The model under review builds one solid part; all positions refer to its coordinate system, in mm. A direction names the side the tool comes from. Round coordinates to 2 decimals unless told otherwise and drop trailing zeros. Write each loop counter-clockwise with the first axis right and the second up, starting at its lowest first coordinate (ties: lowest second). Pieces come first, ordered by that corner, then holes. Notation, with made-up numbers: (61, -36) -> (114, -36) arc R10 ccw to (114, -30) -> close; hole circle Ø11 at (-1.5, 40.5). An arc over 180 degrees is marked (long way). Answer as a JSON object with one key per item and string values. Group by question number.
1) We need section B-B, the plane y = 40.5. Write out the cut boundary in (x, z), then the cut area to 3 significant figures.
2) Mouldability with a two-part tool opening along Y and no side actions: class faces 1 (the flat face through (88, 57.098, 3)), 2 (the flat face through (68, 55, 6)), 3 (the flat face through (107.925, 21.234, 2.958)) as pulls with the +Y half, pulls with the -Y half, needs draft (parallel to the pull), parting line crosses it, or undercut.
3) We need section C-C, the plane z = 3.4. Count the separate pieces of the cut face and the enclosed holes in it, then the cut area to 3 significant figures.
4) Machinability: for faces 4 (the flat face through (27.52, 20.93, 2.96)), 5 (the flat face through (93.83, 73.414, 2.958)), which of the approach directions +Z, -Z, +X, -X, +Y, -Y give a long, thin tool a straight path to every point of the face, cutting with its end or side? Answer none if there is none.
5) To check wall thickness, follow probe 1 along X at (y, z) = (78.5, 3.3); probe 2 along X at (y, z) = (69, 2.8); probe 3 along X at (y, z) = (71, 1.3). State the ranges of each line that lie inside material, in increasing order. Write a range as [from, to].
6) We need section A-A, the plane y = 54. Write out the cut boundary in (x, z).
7) Insertion check: pin 1 Ø1 at (y, z) = (51, 4) entering from -X; pin 2 Ø2.5 at (y, z) = (67.5, 2) entering from -X; pin 3 Ø1.6 at (y, z) = (66.5, 3.5) entering from +X. Each pin has a flat end and moves straight along its axis. Give the tip position at first contact, or say it passes through.
8) We need section D-D, the plane y = 75. Write out the cut boundary in (x, z), then the cut area to 3 significant figures.
from build123d import *

# Parameters (mm, degrees)
MODEL_R             = 3
MODEL_R_2           = 1.5
MODEL_W             = 5.5
MODEL_H             = 5.25
BOSS_EXTRUDE1_DEPTH = 6


with BuildPart() as part:
    # Model → Boss-Extrude1 (new body)
    with BuildSketch(Plane.XY):
        with BuildLine():
            Line((97.092556574, 10.401311798), (38.049140345, 10.401311798))
            Line((38.049140345, 10.401311798), (16.682633066, 31.767819077))
            Line((16.682633066, 31.767819077), (16.576099155, 46.615832828))
            ThreePointArc((16.576099155, 46.615832828), (67.57084846, 98.347641115), (118.565597764, 46.615832828))
            Line((118.565597764, 46.615832828), (118.459063854, 31.767819077))
            Line((118.459063854, 31.767819077), (97.092556574, 10.401311798))
        make_face()
        with Locations((67.57084846, 47.347641115)):
            Circle(MODEL_R, mode=Mode.SUBTRACT)
        with Locations((67.57084846, 57.347641115)):
            Circle(MODEL_R_2, mode=Mode.SUBTRACT)
        with Locations((77.57084846, 47.347641115)):
            Circle(MODEL_R_2, mode=Mode.SUBTRACT)
        with Locations((67.57084846, 37.347641115)):
            Circle(MODEL_R_2, mode=Mode.SUBTRACT)
        with Locations((57.57084846, 47.347641115)):
            Circle(MODEL_R_2, mode=Mode.SUBTRACT)
        Polygon((45.296984853, 69.621504723), (52.191275969, 76.515795839), (48.302188673, 80.404883136), (34.513606439, 66.616300902), (38.402693736, 62.727213606), align=None, mode=Mode.SUBTRACT)
        Polygon((45.296984853, 25.073777508), (52.191275969, 18.179486391), (48.302188673, 14.290399095), (34.513606439, 28.078981328), (38.402693736, 31.968068624), align=None, mode=Mode.SUBTRACT)
        Polygon((89.844712067, 69.621504723), (96.739003184, 62.727213606), (100.62809048, 66.616300902), (86.839508247, 80.404883136), (82.950420951, 76.515795839), align=None, mode=Mode.SUBTRACT)
        Polygon((89.844712067, 25.073777508), (96.739003184, 31.968068624), (100.62809048, 28.078981328), (86.839508247, 14.290399095), (82.950420951, 18.179486391), align=None, mode=Mode.SUBTRACT)
        Polygon((67.57084846, 64.347641115), (72.82084846, 64.347641115), (72.82084846, 69.597641115), (62.32084846, 69.597641115), (62.32084846, 64.347641115), align=None, mode=Mode.SUBTRACT)
        Polygon((36.32084846, 42.347641115), (36.32084846, 45.347641115), (41.82084846, 45.347641115), (41.82084846, 39.347641115), (36.32084846, 39.347641115), align=None, mode=Mode.SUBTRACT)
        Polygon((54.32084846, 42.347641115), (54.32084846, 45.347641115), (48.82084846, 45.347641115), (48.82084846, 39.347641115), (54.32084846, 39.347641115), align=None, mode=Mode.SUBTRACT)
        with Locations((47.57084846, 54.472641115)):
            Rectangle(MODEL_W, MODEL_H, mode=Mode.SUBTRACT)
        Polygon((98.82084846, 42.347641115), (98.82084846, 45.347641115), (93.32084846, 45.347641115), (93.32084846, 39.347641115), (98.82084846, 39.347641115), align=None, mode=Mode.SUBTRACT)
        Polygon((80.82136419, 42.324937285), (80.82136419, 45.324937285), (86.32136419, 45.324937285), (86.32136419, 39.324937285), (80.82136419, 39.324937285), align=None, mode=Mode.SUBTRACT)
        with Locations((87.57084846, 54.472641115)):
            Rectangle(MODEL_W, MODEL_H, mode=Mode.SUBTRACT)
    extrude(amount=BOSS_EXTRUDE1_DEPTH)


solid = part.part
Here are the results:
{
 "1": {"outline": "(16.62, 0) -> (36.32, 0) -> (36.32, 6) -> (16.62, 6) -> close; (41.82, 0) -> (48.82, 0) -> (48.82, 6) -> (41.82, 6) -> close; (54.32, 0) -> (80.82, 0) -> (80.82, 6) -> (54.32, 6) -> close; (86.32, 0) -> (93.32, 0) -> (93.32, 6) -> (86.32, 6) -> close; (98.82, 0) -> (118.52, 0) -> (118.52, 6) -> (98.82, 6) -> close", "area": "479 mm^2"},
 "2": {"face 1": "undercut", "face 2": "needs draft", "face 3": "pulls with the -Y half"},
 "3": {"separate pieces": "1", "enclosed holes": "16", "area": "6,660 mm^2"},
 "4": {"face 4": "+Z, -Z, -X, -Y", "face 5": "+Z, -Z"},
 "5": {"probe 1": "x = [27.19, 46.4], [50.21, 84.93], [88.74, 107.95]", "probe 2": "x = [21.4, 36.9], [44.68, 62.32], [72.82, 90.47], [98.24, 113.75]", "probe 3": "x = [22.39, 38.9], [46.68, 88.47], [96.24, 112.75]"},
 "6": {"outline": "(17.01, 0) -> (44.82, 0) -> (44.82, 6) -> (17.01, 6) -> close; (50.32, 0) -> (84.82, 0) -> (84.82, 6) -> (50.32, 6) -> close; (90.32, 0) -> (118.14, 0) -> (118.14, 6) -> (90.32, 6) -> close"},
 "7": {"pin 1": "stops at x = 16.67", "pin 2": "stops at x = 20.2", "pin 3": "stops at x = 115.15"},
 "8": {"outline": "(24.72, 0) -> (42.9, 0) -> (42.9, 6) -> (24.72, 6) -> close; (50.68, 0) -> (84.47, 0) -> (84.47, 6) -> (50.68, 6) -> close; (92.24, 0) -> (110.42, 0) -> (110.42, 6) -> (92.24, 6) -> close", "area": "421 mm^2"}
}
